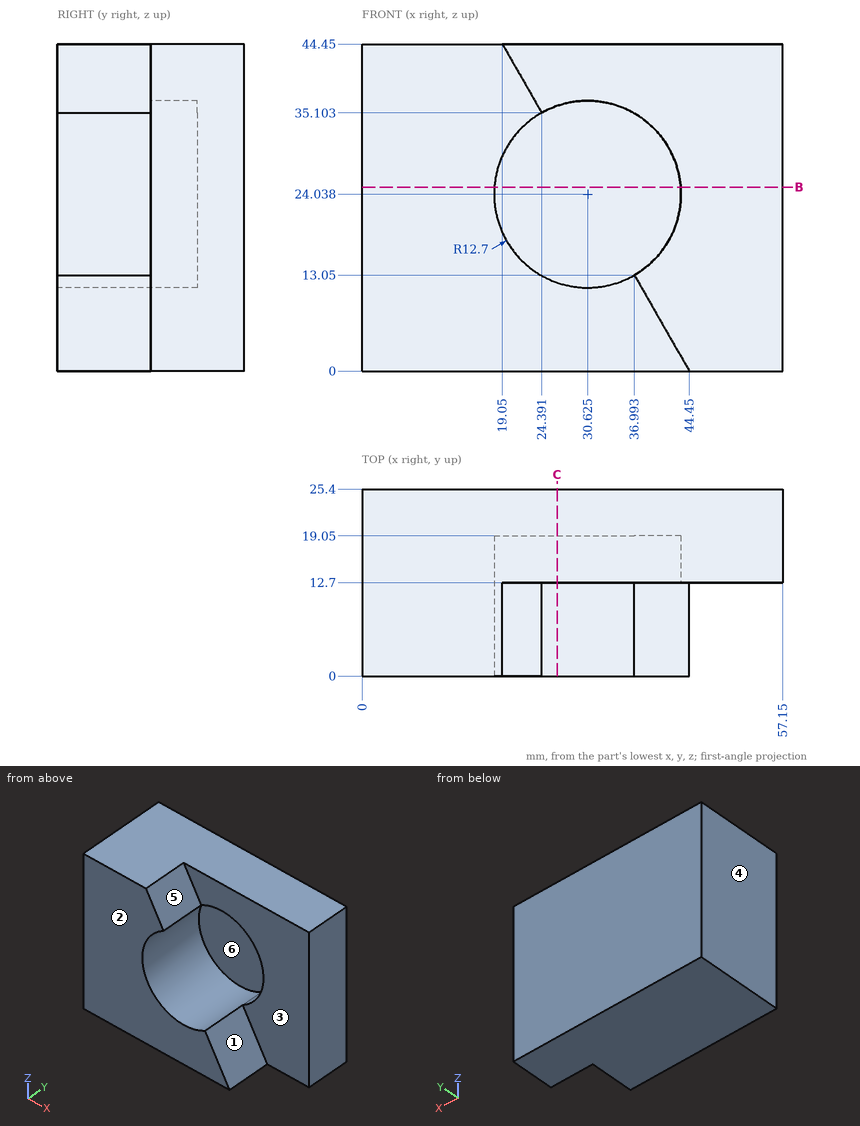
The drawing under review shows one solid part. Ordinate dimensions are in mm from its lowest x, y, z. A direction names the side the tool comes from. Coordinates: 2 decimals unless noted, no trailing zeros. Write each loop counter-clockwise with the first axis right and the second up, starting at its lowest first coordinate (ties: lowest second). Pieces come first, ordered by that corner, then holes. Notation, with made-up numbers: (57, 35.5) - (70, 35.5) arc R10 ccw to (70, 46.5) - close; hole circle Ø3 at (-3, 80). An arc over 180 degrees is marked (long way). Use one line per item in the form item = value.
Q1. The part is to be moulded in two halves that separate along X. For the marked faces 3, 4, 5 and 6, say which applies: +X half, -X half, draft (parallel to the pull), parting line (faces both ways), or undercut.
Taken from the geometry:
face_3 = draft
face_4 = -X half
face_5 = +X half
face_6 = undercut
Q2. Consider section B-B (z = 25). Write out the cut boundary in (x, y), plus the area to 3 significant figures.
Taken from the geometry:
outline = (0, 0) - (17.96, 0) - (17.96, 19.05) - (43.29, 19.05) - (43.29, 12.7) - (57.15, 12.7) - (57.15, 25.4) - (0, 25.4) - close
area = 793 mm^2
Q3. For probe 1 along X at (y, z) = (15.75, 30); probe 2 along Y at (x, z) = (24.5, 16); probe 3 along Y at (x, z) = (42, 39.5), list the stretches that pass through material, from the lowest coordinate up.
Taken from the geometry:
probe_1 = 0 to 19.41, 41.84 to 57.15
probe_2 = 19.05 to 25.4
probe_3 = 12.7 to 25.4
Q4. Insertion check: pin 1 Ø3 at (y, z) = (11.5, 17.5) entering from +X; pin 2 Ø1.5 at (x, y) = (41, 3) entering from +Z. Each pin has a flat end and moves straight along its axis. Give the tip position at first contact, or say it passes through.
Taken from the geometry:
pin_1 = 57.15
pin_2 = 7.35
Q5. Consider section C-C (x = 26.5). Write out the cut boundary in (y, z), plus the area to 3 significant figures.
Taken from the geometry:
outline = (0, 0) - (25.4, 0) - (25.4, 44.45) - (12.7, 44.45) - (12.7, 36.05) - (19.05, 36.05) - (19.05, 12.03) - (0, 12.03) - close
area = 565 mm^2
Q6. Machinability: for the marked faces 1 and 2, which of the approach directions +Z, -Z, +X, -X, +Y, -Y give a long, thin tool a straight path to every point of the face, cutting with its end or side? Answer none if there is none.
Taken from the geometry:
face_1 = +Z, +X, -Y
face_2 = +Z, -Z, +X, -X, -Y
